Autodesk Inventor part; units mm, degrees
ref_plane "YZ Plane" through (0, 0, 0) normal (1, 0, 0) x (0, 1, 0)
ref_plane "XZ Plane" through (0, 0, 0) normal (0, 1, 0) x (-1, 0, 0)
ref_plane "XY Plane" through (0, 0, 0) normal (0, 0, 1) x (1, 0, 0)
sketch "Sketch1" plane through (0, 0, 0) normal (0, 0, 1) x (1, 0, 0)
  line L0 (0, 0) -> (175, 0)
  line L1 (175, 0) -> (175, 91.44)
  line L2 (175, 91.44) -> (76.7273, 91.44)
  line L3 (76.7273, 91.44) -> (0, 0)
  dimension "d0" = 175
  dimension "d1" = 91.44
  dimension "d101" = 50
extrude "Extrusion1" add sketch "Sketch1" along normal blind 9.525
sketch "Sketch11" plane through (0, 0, 0) normal (0, 0, -1) x (-1, 0, 0)
  circle A0 centre (-106.6758, 11.5887) radius 6.35
  circle A1 centre (-106.6758, 11.5887) radius 6.9469
  dimension "d121" = 12.7
  dimension "d122" = 13.8938
sketch "Sketch8" plane through (0, 0, 0) normal (0, 0, -1) x (-1, 0, 0)
  circle A0 centre (-73.1284, 38.046) radius 7
  dimension "d105" = 14
sketch "Sketch9" plane through (0, 0, 0) normal (0, 0, -1) x (-1, 0, 0)
  circle A0 centre (-85.6284, 38.046) radius 1.25
  circle A1 centre (-60.6284, 38.046) radius 1.25
extrude "Extrusion2" cut sketch "Sketch8" against normal blind 9.525
hole "Hole7" at (85.6284, 38.046, 0) at (60.6284, 38.046, 0) direction (0, 0, 1) diameter 3.4036 end through all
sketch "Sketch10" plane through (0, 0, 0) normal (0, 0, -1) x (-1, 0, 0)
  circle A0 centre (-106.6758, 31.4833) radius 6.35
  dimension "d118" = 12.7
extrude "Extrusion3" cut sketch "Sketch10" against normal blind 9.525
extrude "Extrusion4" cut sketch "Sketch11" against normal blind 9.525 contours A0
sketch "Sketch12" plane through (0, 0, 0) normal (0, -1, 0) x (1, 0, 0)
  line L0 (175, 9.525) -> (0, 9.525)
  line L1 (0, 0) -> (175, 0)
  line L2 (33.02, 9.525) -> (80.01, 9.525)
  line L3 (80.01, 9.525) -> (80.01, 0)
  line L4 (80.01, 0) -> (33.02, 0)
  line L5 (33.02, 0) -> (33.02, 9.525)
  line L6 (175, 0) -> (175, 9.525)
  dimension "d126" = 46.99
  dimension "d196" = 94.99
extrude "Extrusion5" cut sketch "Sketch12" against normal blind 16.51 contours L3 L1 L5 L0
sketch "Sketch13" plane through (76.7273, 91.44, 0) normal (0, 1, 0) x (1, 0, 0)
  line L0 (98.2727, 0) -> (0, 0)
  line L1 (61.4427, 0) -> (98.2727, 0)
  line L2 (98.2727, 0) -> (98.2727, -9.525)
  line L3 (98.2727, -9.525) -> (61.4427, -9.525)
  line L4 (61.4427, -9.525) -> (61.4427, 0)
  point P0 (-76.7273, 0)
  dimension "d129" = 36.83
extrude "Extrusion6" cut sketch "Sketch13" against normal blind 50.8
sketch "Sketch14" plane through (76.7273, 91.44, 9.525) normal (0, 1, 0) x (1, 0, 0)
  line L0 (0, 9.525) -> (0, 0)
  line L1 (-76.7273, 0) -> (0, 0)
  line L2 (0, 9.525) -> (0, 0)
  line L3 (0, 9.525) -> (-76.7273, 9.525)
  line L4 (-76.7273, 9.525) -> (-76.7273, 0)
  line L5 (-24.13, 9.525) -> (-125.73, 9.525)
  line L6 (-125.73, 9.525) -> (-125.73, 0)
  line L7 (-125.73, 0) -> (-24.13, 0)
  line L8 (-24.13, 0) -> (-24.13, 9.525)
  dimension "d132" = 24.13
  dimension "d133" = 101.6
extrude "Extrusion7" cut sketch "Sketch14" against normal blind 62.992 contours L8 L1 L4 L3 | L4 L7 L6 L5
sketch "Sketch15" plane through (76.7273, 91.44, 9.525) normal (0, 1, 0) x (1, 0, 0)
  line L0 (61.4427, 9.525) -> (0, 9.525)
  line L1 (0, 9.525) -> (0, 0)
  line L2 (0, 0) -> (61.4427, 0)
  line L3 (38.1, 9.525) -> (47.625, 9.525)
  line L4 (47.625, 9.525) -> (47.625, 0)
  line L5 (47.625, 0) -> (38.1, 0)
  line L6 (38.1, 0) -> (38.1, 9.525)
  point P0 (-76.7273, 9.525)
  dimension "d136" = 9.525
  dimension "d137" = 38.1
extrude "Extrusion8" cut sketch "Sketch15" against normal blind 9.525 contours L4 L2 L6 L0
sketch "Sketch16" plane through (175, 0, 0) normal (0, -1, 0) x (1, 0, 0)
  line L0 (-94.99, 0) -> (0, 0)
  line L1 (0, 0) -> (0, 9.525)
  line L2 (0, 9.525) -> (-94.99, 9.525)
  line L3 (-47.625, 9.525) -> (-38.1, 9.525)
  line L4 (-38.1, 9.525) -> (-38.1, 0)
  line L5 (-38.1, 0) -> (-47.625, 0)
  line L6 (-47.625, 0) -> (-47.625, 9.525)
  point P0 (-175, 0)
  dimension "d140" = 38.1
  dimension "d141" = 9.525
extrude "Extrusion9" cut sketch "Sketch16" against normal blind 9.525 contours L6 L2 L4 L0
sketch "Sketch17" plane through (76.7273, 81.915, 9.525) normal (0, 1, 0) x (1, 0, 0)
  circle A0 centre (42.8625, 4.7625) radius 2.2479
  point P0 (-76.7273, 9.525)
hole "Hole8" at (119.5898, 81.915, 4.7625) direction (0, -1, 0) diameter 3.302 depth 12.7 tip angle 118
sketch "Sketch18" plane through (175, 9.525, 0) normal (0, -1, 0) x (1, 0, 0)
  circle A0 centre (-42.8625, 4.7625) radius 2.2479
  point P0 (-175, 0)
hole "Hole9" at (132.1375, 9.525, 4.7625) direction (0, 1, 0) diameter 3.302 depth 12.7 tip angle 118
sketch "Sketch19" plane through (76.7273, 40.64, 0) normal (0, 1, 0) x (1, 0, 0)
  circle A0 centre (71.6027, -4.7625) radius 2.2479
  circle A1 centre (89.3827, -4.7625) radius 2.2479
  point P0 (-76.7273, 0)
hole "Hole10" at (148.33, 40.64, 4.7625) at (166.11, 40.64, 4.7625) direction (0, -1, 0) diameter 3.302 depth 12.7 tip angle 118
sketch "Sketch20" plane through (175, 0, 9.525) normal (1, 0, 0) x (0, 0, -1)
  line L0 (9.525, 40.64) -> (0, 40.64)
  line L1 (9.525, 0) -> (0, 0)
  point P0 (4.7625, 10.16)
  point P1 (4.7625, 30.48)
  dimension "d165" = 30.48
  dimension "d166" = 10.16
  dimension "d167" = 10.16
hole "Hole11" at (175, 10.16, 4.7625) at (175, 30.48, 4.7625) direction (-1, 0, 0) diameter 3.302 depth 12.7 tip angle 118
sketch "Sketch21" plane through (52.5973, 28.448, 0) normal (-1, 0, 0) x (0, 0, 1)
  circle A0 centre (3.79, 4.06) radius 1.0795
  circle A1 centre (3.79, 4.06) radius 1.55
  circle A2 centre (44.49, 20.36) radius 1.55
  line L0 (46.99, 22.86) -> (46.99, 1.56)
  line L1 (1.29, 22.86) -> (46.99, 22.86)
  line L2 (1.29, 1.56) -> (1.29, 22.86)
  line L3 (46.99, 1.56) -> (1.29, 1.56)
  line L4 (1.29, 12.21) -> (46.99, 12.21)
  circle A3 centre (3.79, 20.36) radius 1.0795
  point P0 (0, -28.448)
hole "Hole12" at (52.5973, 48.808, 3.79) at (52.5973, 32.508, 3.79) direction (1, 0, 0) diameter 2.159 depth 5.08 tip angle 118
sketch "Sketch22" plane through (76.7273, 91.44, 0) normal (-0.7660444, 0.6427876, 0) x (0, 0, 1)
  circle A0 centre (4.7625, -7.62) radius 2.159
  circle A1 centre (4.7625, -33.02) radius 2.159
  circle A2 centre (4.7625, -84.7725) radius 2.2479
  point P0 (0, -119.3664)
hole "Hole13" at (71.8292, 85.6027, 4.7625) at (55.5024, 66.1452, 4.7625) at (22.2366, 26.5005, 4.7625) direction (0.7660444, -0.6427876, 0) diameter 3.302 depth 5.08 tip angle 118
sketch "Sketch23" plane through (0, 0, 0) normal (-0.7660444, 0.6427876, 0) x (0, 0, 1)
  circle A0 centre (4.7625, 24.1164) radius 2.159
hole "Hole14" at (15.5018, 18.4743, 4.7625) direction (0.7660444, -0.6427876, 0) diameter 3.302 depth 7.62 tip angle 118
properties part number "Inside Chassis3" material "Aluminum-6061"
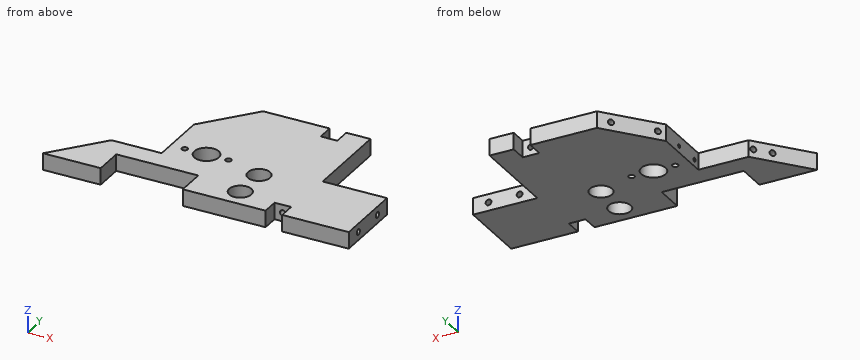
CAD build for the part. Positions are in the model's coordinates, mm. Coordinates: 2 decimals unless noted, no trailing zeros. Order: outer loops, then holes, each group sorted by start corner. A loop starts at its lowest first (then second) coordinate and runs counter-clockwise, first axis right, second up. Notation, with made-up numbers: (19.5, 29.25) - (40.5, 29.25) arc R24 ccw to (40.5, 62.25) - close; hole circle Ø1 at (51.25, 41). An arc over 180 degrees is marked (long way). Answer in a Markdown table with one row per item.
1. Drill centre lines: L1, parallel to X at y = 32, z = 1.25; L2, parallel to X at y = 30, z = 5.5; L3, parallel to X at y = 32, z = 6. Where is each one in solid material? Low to high. Write a range as from..to.
Answer:
| item | result |
|---|---|
| L1 | 52.6..69.6, 76.66..100.35, 113..175 |
| L2 | 52.6..100.5, 112.85..146.85, 149.81..161.84 |
| L3 | 52.6..69.6, 76.66..100.35, 113..147.24, 149.42..165.02, 167.2..175 |
2. Flat gauge pins, fed straight in: P1, Ø2, axis at y = 45, z = 5, coming from the +X side; P2, Ø2, axis at y = 30.48, z = 4.76, coming from the +X side; P3, Ø4, axis at y = 43.5, z = 6.5, coming from the -X side; P4, Ø12.5, axis at x = 73.13, y = 38.05, coming from the +Z side. Where does each tip first touch, or does it go through?
Answer:
| item | result |
|---|---|
| P1 | x = 138.17 |
| P2 | x = 161.91 |
| P3 | x = 52.6 |
| P4 | through |
3. Slice it at C-C, the plane x = 30. List the corners of the cut face in (y, z) (3 decimals).
Answer:
| item | result |
|---|---|
| outline | (0, 0) - (28.448, 0) - (28.448, 9.525) - (0, 9.525) - close |
4. Slice it at A-A, the plane x = 106.5. List the corners of the cut face in (y, z) (3 decimals).
Answer:
| item | result |
|---|---|
| outline | (0, 0) - (5.241, 0) - (5.241, 9.525) - (0, 9.525) - close; (17.936, 0) - (25.136, 0) - (25.136, 9.525) - (17.936, 9.525) - close; (37.831, 0) - (91.44, 0) - (91.44, 9.525) - (37.831, 9.525) - close |
5. Slice it at B-B, the plane y = 58. List the corners of the cut face in (x, z) (3 decimals), then the cut area to 3 significant figures.
Answer:
| item | result |
|---|---|
| outline | (52.597, 0) - (138.17, 0) - (138.17, 9.525) - (52.597, 9.525) - close |
| area | 815 mm² |
